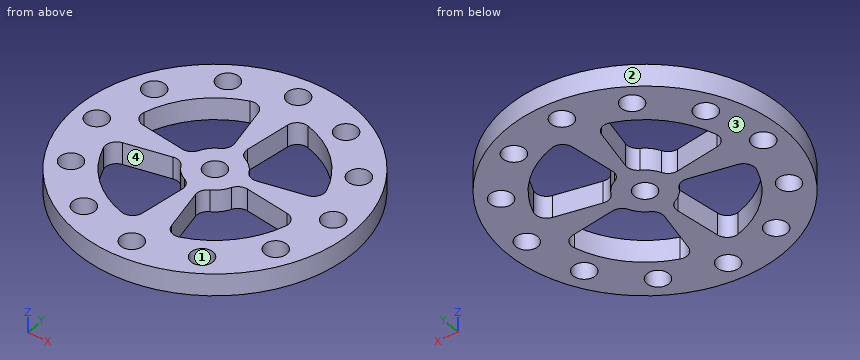
```python
from build123d import *

# Parameters (mm, degrees)
F0_R     = 25
F0_R_2   = 2
F1_DEPTH = 4
F3_DEPTH = 25
F4_DEPTH = 25


# Not quite as in the source:
# - a feature names something its author has since deleted; it is built from what else it names


with BuildPart() as f1:
    # F0 (on Top) → F1 (new body)
    with BuildSketch(Plane.XY):
        Circle(F0_R)
        with Locations((-10.5, -18.1865334795)):
            Circle(F0_R_2, mode=Mode.SUBTRACT)
        with Locations((-18.1865334795, -10.5)):
            Circle(F0_R_2, mode=Mode.SUBTRACT)
        with Locations((0, -21)):
            Circle(F0_R_2, mode=Mode.SUBTRACT)
        with Locations((10.5, -18.1865334795)):
            Circle(F0_R_2, mode=Mode.SUBTRACT)
        with Locations((18.1865334795, -10.5)):
            Circle(F0_R_2, mode=Mode.SUBTRACT)
        with Locations((-21, 0)):
            Circle(F0_R_2, mode=Mode.SUBTRACT)
        with Locations((-18.1865334795, 10.5)):
            Circle(F0_R_2, mode=Mode.SUBTRACT)
        with Locations((-10.5, 18.1865334795)):
            Circle(F0_R_2, mode=Mode.SUBTRACT)
        Circle(F0_R_2, mode=Mode.SUBTRACT)
        with Locations((21, 0)):
            Circle(F0_R_2, mode=Mode.SUBTRACT)
        with Locations((18.1865334795, 10.5)):
            Circle(F0_R_2, mode=Mode.SUBTRACT)
        with Locations((10.5, 18.1865334795)):
            Circle(F0_R_2, mode=Mode.SUBTRACT)
        with Locations((0, 21)):
            Circle(F0_R_2, mode=Mode.SUBTRACT)
    extrude(amount=-F1_DEPTH)

    # F2 (on face) → F3 (cut)
    with BuildSketch(Plane.XY):
        with BuildLine():
            ThreePointArc((4.470710633, 2.2389163531), (5.3603810508, 1.3477279657), (6.6062912415, 1.1648673883))
            Line((6.6062912415, 1.1648673883), (14.6402197592, 2.581465747))
            ThreePointArc((14.6402197592, 2.581465747), (16.0042145423, 3.5159567971), (16.1986465243, 5.1578920868))
            ThreePointArc((16.1986465243, 5.1578920868), (12.0208152802, 12.0208152802), (5.1578920868, 16.1986465243))
            ThreePointArc((5.1578920868, 16.1986465243), (3.5159567971, 16.0042145423), (2.581465747, 14.6402197592))
            Line((2.581465747, 14.6402197592), (1.1648673883, 6.6062912415))
            ThreePointArc((1.1648673883, 6.6062912415), (1.3477279657, 5.3603810508), (2.2389163531, 4.470710633))
            ThreePointArc((2.2389163531, 4.470710633), (3.5355339059, 3.5355339059), (4.470710633, 2.2389163531))
        make_face()
        with BuildLine():
            ThreePointArc((-4.470710633, -2.2389163531), (-5.3603810508, -1.3477279657), (-6.6062912415, -1.1648673883))
            Line((-6.6062912415, -1.1648673883), (-14.6402197592, -2.581465747))
            ThreePointArc((-14.6402197592, -2.581465747), (-16.0042145423, -3.5159567971), (-16.1986465243, -5.1578920868))
            ThreePointArc((-16.1986465243, -5.1578920868), (-12.0208152802, -12.0208152802), (-5.1578920868, -16.1986465243))
            ThreePointArc((-5.1578920868, -16.1986465243), (-3.5159567971, -16.0042145423), (-2.581465747, -14.6402197592))
            Line((-2.581465747, -14.6402197592), (-1.1648673883, -6.6062912415))
            ThreePointArc((-1.1648673883, -6.6062912415), (-1.3477279657, -5.3603810508), (-2.2389163531, -4.470710633))
            ThreePointArc((-2.2389163531, -4.470710633), (-3.5355339059, -3.5355339059), (-4.470710633, -2.2389163531))
        make_face()
        with BuildLine():
            ThreePointArc((2.2389163531, -4.470710633), (1.3477279657, -5.3603810508), (1.1648673883, -6.6062912415))
            Line((1.1648673883, -6.6062912415), (2.581465747, -14.6402197592))
            ThreePointArc((2.581465747, -14.6402197592), (3.5159567971, -16.0042145423), (5.1578920868, -16.1986465243))
            ThreePointArc((5.1578920868, -16.1986465243), (12.0208152802, -12.0208152802), (16.1986465243, -5.1578920868))
            ThreePointArc((16.1986465243, -5.1578920868), (16.0042145423, -3.5159567971), (14.6402197592, -2.581465747))
            Line((14.6402197592, -2.581465747), (6.6062912415, -1.1648673883))
            ThreePointArc((6.6062912415, -1.1648673883), (5.3603810508, -1.3477279657), (4.470710633, -2.2389163531))
            ThreePointArc((4.470710633, -2.2389163531), (3.5355339059, -3.5355339059), (2.2389163531, -4.470710633))
        make_face()
    extrude(amount=-F3_DEPTH, mode=Mode.SUBTRACT)

    # F2 (on face) → F4 (cut)
    with BuildSketch(Plane.XY):
        with BuildLine():
            ThreePointArc((-2.581465747, 14.6402197592), (-3.5159567971, 16.0042145423), (-5.1578920868, 16.1986465243))
            ThreePointArc((-5.1578920868, 16.1986465243), (-12.0208152802, 12.0208152802), (-16.1986465243, 5.1578920868))
            ThreePointArc((-16.1986465243, 5.1578920868), (-16.0042145423, 3.5159567971), (-14.6402197592, 2.581465747))
            Line((-14.6402197592, 2.581465747), (-6.6062912415, 1.1648673883))
            ThreePointArc((-6.6062912415, 1.1648673883), (-5.3603810508, 1.3477279657), (-4.470710633, 2.2389163531))
            ThreePointArc((-4.470710633, 2.2389163531), (-3.5355339059, 3.5355339059), (-2.2389163531, 4.470710633))
            ThreePointArc((-2.2389163531, 4.470710633), (-1.3477279657, 5.3603810508), (-1.1648673883, 6.6062912415))
            Line((-1.1648673883, 6.6062912415), (-2.581465747, 14.6402197592))
        make_face()
    extrude(amount=-F4_DEPTH, mode=Mode.SUBTRACT)


solid = f1.part
```
Geometry check sheet. Reference: the model listing, model coordinates, mm. Face numbers are marked on the shaded views. Give positions to 0.01 mm unless a question says otherwise; leave off trailing zeros. Write each loop counter-clockwise with the first axis right and the second up, starting at its lowest first coordinate (ties: lowest second). Pieces come first, ordered by that corner, then holes.
1) Section check C-C, the plane x = 11. Record the boundary of the cut face in (y, z), and give its area (3 significant figures).
2) Release check for a two-part mould opening along Y. For the marked faces 1, 2, 3 and 4 record: pulls with the +Y half, pulls with the -Y half, needs draft (parallel to the pull), parting line crosses it, or undercut.
3) Section check D-D, the plane y = -21. Record the boundary of the cut face in (x, z), and give its area (3 significant figures).
4) Material ranges on L1, parallel to Y at x = 0, z = -2.5; L2, parallel to Y at x = -3, z = -0.9; L3, parallel to Y at x = -5, z = -1.85, recorded low to high.
5) Gauge pin test, flat end, axial feed: pin 1 (1.5 mm diameter, centred on y = 8, z = -2, fed in from +X). Record the tip position at first contact, or that the pin passes through.
6) Section check A-A, the plane y = 0. Record the boundary of the cut face in (x, z).
Computed:
1. outline: (-22.45, -4) - (-20.12, -4) - (-20.12, 0) - (-22.45, 0) - close; (-16.25, -4) - (-12.96, -4) - (-12.96, 0) - (-16.25, 0) - close; (-1.94, -4) - (1.94, -4) - (1.94, 0) - (-1.94, 0) - close; (12.96, -4) - (16.25, -4) - (16.25, 0) - (12.96, 0) - close; (20.12, -4) - (22.45, -4) - (22.45, 0) - (20.12, 0) - close
1. area: 60.4 mm2
2. face 1: undercut
2. face 2: parting line crosses it
2. face 3: needs draft
2. face 4: undercut
3. outline: (-13.56, -4) - (-2, -4) - (-2, 0) - (-13.56, 0) - close; (2, -4) - (13.56, -4) - (13.56, 0) - (2, 0) - close
3. area: 92.5 mm2
4. L1: y = -25 to -23, -19 to -2, 2 to 19, 23 to 25
4. L2: y = -24.82 to -15.56, -4 to 4, 15.56 to 24.82
4. L3: y = -24.49 to -16.24, -1.58 to 1.58, 16.24 to 24.49
5. pin 1: stops at x = 23.93
6. outline: (-25, -4) - (-23, -4) - (-23, 0) - (-25, 0) - close; (-19, -4) - (-2, -4) - (-2, 0) - (-19, 0) - close; (2, -4) - (19, -4) - (19, 0) - (2, 0) - close; (23, -4) - (25, -4) - (25, 0) - (23, 0) - close
